Autodesk Inventor part; units mm, degrees
ref_plane "YZ Plane" through (0, 0, 0) normal (1, 0, 0) x (0, 1, 0)
ref_plane "XZ Plane" through (0, 0, 0) normal (0, 1, 0) x (-1, 0, 0)
ref_plane "XY Plane" through (0, 0, 0) normal (0, 0, 1) x (1, 0, 0)
sketch "Sketch1" plane through (0, 0, 0) normal (0, 0, 1) x (1, 0, 0)
  line L0 (0, 0) -> (25, 0)
  line L1 (25, 0) -> (25, 10)
  line L2 (25, 10) -> (0, 10)
  line L3 (0, 10) -> (0, 0)
  dimension "d0" = 25
  dimension "d1" = 10
extrude "Extrusion1" add sketch "Sketch1" along normal blind 15
sketch "Sketch2" plane through (0, 0, 15) normal (0, 0, 1) x (1, 0, 0)
  circle A0 centre (20, 5) radius 3
  point P0 (0, 0)
  dimension "d4" = 6
extrude "Extrusion2" add sketch "Sketch2" along normal blind 5
sketch "Sketch3" plane through (20, 5, 20) normal (0, 0, 1) x (1, 0, 0)
  circle A0 centre (0, 0) radius 1.5
  point P0 (-20, -5)
  dimension "d7" = 3
extrude "Extrusion3" cut sketch "Sketch3" against normal blind 3
sketch "Sketch4" plane through (20, 5, 20) normal (0, 0, 1) x (1, 0, 0)
  circle A0 centre (0, 0) radius 3
  point P0 (-20, -5)
extrude "Extrusion4" add sketch "Sketch4" along normal blind 9
sketch "Sketch5" plane through (20, 5, 29) normal (0, 0, 1) x (1, 0, 0)
  circle A0 centre (0, 0) radius 1.5
  circle A1 centre (0, 0) radius 1.5
  point P0 (-20, -5)
extrude "Extrusion5" cut sketch "Sketch5" against normal blind 5
properties part number "servo part"
Input: part model. Units: mm. Frame: model coordinates. A direction names the side the tool comes from. Coordinates: 2 decimals unless noted, no trailing zeros. Loops run counter-clockwise (first coordinate to the right, second up) from the corner with the lowest first, then second, coordinate; pieces in that order, holes last. Notation, with made-up numbers: (53.25, 80.5) - (100.25, 80.5) arc R11 cw to (100.25, 101.5) - close; hole circle Ø5 at (44, -26.5). An arc over 180 degrees is marked (long way). Answer in a Markdown table with one row per item.
(1) Cut plane A-A on y = 5. Output: boundary loops of the cut face in (x, z), plus the area to 3 significant figures.
Model answer:
| item | result |
|---|---|
| outline | (0, 0) - (25, 0) - (25, 15) - (23, 15) - (23, 29) - (21.5, 29) - (21.5, 24) - (18.5, 24) - (18.5, 29) - (17, 29) - (17, 15) - (0, 15) - close; hole (18.5, 17) - (21.5, 17) - (21.5, 20) - (18.5, 20) - close |
| area | 435 mm² |
(2) Mould query, pull axis X, two halves, no side actions, for faces 1 (the face through (25, 5, 7)), 2 (the face through (12, 5, 0)), 3 (the face through (20, 5, 20)), 4 (the face through (17.79, 2.97, 21.9)). Classes: pulls with the +X half, pulls with the -X half, needs draft (parallel to the pull), parting line crosses it, or undercut.
Model answer:
| item | result |
|---|---|
| face 1 | pulls with the +X half |
| face 2 | needs draft |
| face 3 | undercut |
| face 4 | parting line crosses it |
(3) Pin query (flat end, axial travel): P1, Ø3, axis at y = 2.5, z = 18.5, coming from the -X side; P2, Ø3, axis at x = 11, y = 2.5, coming from the +Z side; P3, Ø0.9, axis at x = 20.5, y = 5, coming from the +Z side. Return the tip coordinate at first contact, or that it passes through.
Model answer:
| item | result |
|---|---|
| P1 | stops at x = 17.17 |
| P2 | stops at z = 15 |
| P3 | stops at z = 24 |
(4) Material intervals for L1, parallel to Y at x = 20, z = 26.05; L2, parallel to Z at x = 16.75, y = 1; L3, parallel to Z at x = 19.5, y = 5, sorted ascending. Write a range as from..to.
Model answer:
| item | result |
|---|---|
| L1 | y = 2..3.5, 6.5..8 |
| L2 | z = 0..15 |
| L3 | z = 0..17, 20..24 |
(5) Cut plane B-B on x = 20. Output: boundary loops of the cut face in (y, z).
Model answer:
| item | result |
|---|---|
| outline | (0, 0) - (10, 0) - (10, 15) - (8, 15) - (8, 29) - (6.5, 29) - (6.5, 24) - (3.5, 24) - (3.5, 29) - (2, 29) - (2, 15) - (0, 15) - close; hole (3.5, 17) - (6.5, 17) - (6.5, 20) - (3.5, 20) - close |
(6) Cut plane C-C on z = 18.5. Output: boundary loops of the cut face in (x, y), plus the area to 3 significant figures.
Model answer:
| item | result |
|---|---|
| outline | circle Ø6 at (20, 5); hole circle Ø3 at (20, 5) |
| area | 21.2 mm² |
(7) Cut plane D-D on z = 23.5. Output: boundary loops of the cut face in (x, y).
Model answer:
| item | result |
|---|---|
| outline | circle Ø6 at (20, 5) |
(8) Set-up query: faces 5 (the face through (12, 0, 7)), 6 (the face through (20, 5, 24)), 7 (the face through (18.5, 5.07, 18.52)). Return all of +Z, -Z, +X, -X, +Y, -Y with unobstructed straight access to the full face (end or side cutting, diameter ignored); none if empty.
Model answer:
| item | result |
|---|---|
| face 5 | +Z, -Z, +X, -X, -Y |
| face 6 | +Z |
| face 7 | none |
